The model under review builds one solid part; all positions refer to its coordinate system, in mm. A direction names the side the tool comes from. Give positions to 0.01 mm unless a question says otherwise; leave off trailing zeros. Loops run counter-clockwise (first coordinate to the right, second up) from the corner with the lowest first, then second, coordinate; pieces in that order, holes last. Notation, with made-up numbers: M 12,60 L 27,60 A20 cw 27,73 Z; hole C 29,52 d9. An arc over 180 degrees is marked long. One line per item, written item: value. Start each with the question number.
Q1. We need section C-C on z = -2.75. Write out the cut boundary in (x, y), plus the area to 3 significant figures.
Q2. We need section B-B on x = -21. Write out the cut boundary in (y, z).
Q3. For faces 1 (the face through (-19.8, 7.6, -5)), 2 (the face through (8.834, 10.14, -16.465)), 3 (the face through (15, 10, -10)), 4 (the face through (0, 0, -6)), 5 (the face through (27, 10, -2)), list the 3-axis set-ups (+Z, -Z, +X, -X, +Y, -Y) from which the entire face can be reached by the end or side of a thin tool; tool diameter is ignored.
Q4. We need section D-D on y = 2.5. Write out the cut boundary in (x, z), plus the area to 3 significant figures.
Q5. To check wall thickness, follow line 1 along Y through (x, z) = (21, -2.1); line 2 along X through (y, z) = (11, -4); line 3 along Z through (x, y) = (-19, 15.75). State the ranges of each line that lie inside material, in increasing order. Write a range as from..to.
Q6. We need section A-A on y = 10. Write out the cut boundary in (x, z), plus the area to 3 significant figures.
Q7. Mouldability with a two-part tool opening along X and no side actions: class faces 6 (the face through (11, 10, -16.642)), 7 (the face through (-15, 10, -10)), 8 (the face through (23, 8.5, -2.5)) as released by +X, released by -X, zero draft, split by the parting line, or undercut.
Q8. For pin 1 (2 mm diameter, centred on x = 21.5, y = 13, fed in from -Z); pin 2 (1 mm diameter, centred on x = -8.5, y = 15.5, fed in from -Z); pin 3 (8.5 mm diameter, centred on y = 6, z = -11.5, fed in from +X); pin 4 (10 mm diameter, centred on x = 6.5, y = 15.5, fed in from +Z), all flat-tipped, find the tip position at first contact; note any pin that passes through.
Autodesk Inventor part; units mm, degrees
ref_plane "YZ Plane" through (0, 0, 0) normal (1, 0, 0) x (0, 1, 0)
ref_plane "XZ Plane" through (0, 0, 0) normal (0, 1, 0) x (-1, 0, 0)
ref_plane "XY Plane" through (0, 0, 0) normal (0, 0, 1) x (1, 0, 0)
sketch "Sketch1" plane through (0, 0, 0) normal (0, 1, 0) x (-1, 0, 0)
  circle A0 centre (0, -19.05) radius 9
  line L0 (15, 0) -> (-15, 0)
  line L1 (-15, 0) -> (-15, -16.6415)
  line L2 (-15, -16.6415) -> (15, -16.6415)
  line L3 (15, -16.6415) -> (15, 0)
  line L4 (-27, -5) -> (27, -5)
  line L5 (27, -5) -> (27, 0)
  line L6 (27, 0) -> (-27, 0)
  line L7 (-27, 0) -> (-27, -5)
  line L8 (-27, -5) -> (27, 0) construction
  line L9 (27, -5) -> (-27, 0) construction
  point P0 (0, 0)
  point P1 (0, -2.5)
  point P2 (0, -2.5)
  point P3 (0, -2.5)
  point P4 (15, -5)
  point P5 (15, 0)
  point P6 (-15, -5)
  point P7 (-15, 0)
  point P8 (0, 0)
  dimension "d0" = 18
  dimension "d1" = 19.05
  dimension "d5" = 15
  dimension "d6" = 15
  dimension "d7" = 27
  dimension "d13" = 5
extrude "Extrusion1" add sketch "Sketch1" along normal blind 20 contours A0 L2 L1 L4 L3 | L4 L1 L0 L3 | L3 L6 L5 L4 | L4 L7 L6 L1
sketch "Sketch2" plane through (27, 0, -5) normal (0, 0, -1) x (-1, 0, 0)
  circle A0 centre (6, 10) radius 2.5
  line L0 (0, 0) -> (0, 20)
  line L1 (0, 20) -> (12, 20)
  point P0 (27, 0)
  point P1 (6, 20)
  dimension "d10" = 6
  dimension "d11" = 10
  dimension "d12" = 5
extrude "Extrusion2" cut sketch "Sketch2" against normal through all
mirror "Mirror1" about plane through (0, 0, 0) normal (1, 0, 0) of "Extrusion2"
fillet "Fillet2" radius 1 2 edges at (8.6718, 10, -16.6415) (-8.6718, 10, -16.6415)
fillet "Fillet3" radius 1 2 edges at (27, 10, -5) (-27, 10, -5)
sketch "Sketch3" plane through (-15, 0, -5) normal (0, 0, -1) x (-1, 0, 0)
  circle A0 centre (6, 10) radius 2.5
  circle A1 centre (6, 10) radius 5
  line L0 (11, 20) -> (11, 0)
  point P0 (-15, 0)
fillet "Fillet4" radius 1 2 edges at (15, 10, -5) (-15, 10, -5)
fillet "Fillet5" radius 3 2 edges at (15, 10, -16.6415) (-15, 10, -16.6415)
properties part number "Shaft support"
Solved:
1. outline: M -27,0 L 27,0 L 27,20 L -27,20 Z; hole C -21,10 d5; hole C 21,10 d5
1. area: 1,040 mm2
2. outline: M 0,-5 L 7.5,-5 L 7.5,0 L 0,0 Z; M 12.5,-5 L 20,-5 L 20,0 L 12.5,0 Z
3. face 1: -Z, -X, +Y, -Y
3. face 2: -Z, +Y, -Y
3. face 3: -Z, +X, +Y, -Y
3. face 4: +Z, -Z, +X, -X, -Y
3. face 5: +Z, -Z, +X, +Y, -Y
4. outline: M -27,-4 A1 ccw -26,-5 L -16,-5 A1 cw -15,-6 L -15,-13.64 A3 ccw -12,-16.64 L -9.4,-16.64 A1 ccw -8.46,-15.98 A9 cw 8.46,-15.98 A1 ccw 9.4,-16.64 L 12,-16.64 A3 ccw 15,-13.64 L 15,-6 A1 cw 16,-5 L 26,-5 A1 ccw 27,-4 L 27,0 L -27,0 Z
4. area: 531 mm2
5. line 1: 0..7.5, 12.5..20
5. line 2: -27..-23.29, -18.71..18.71, 23.29..27
5. line 3: -5..0
6. outline: M -27,-4 A1 ccw -26,-5 L -23.5,-5 L -23.5,0 L -27,0 Z; M -18.5,-5 L -16,-5 A1 cw -15,-6 L -15,-13.64 A3 ccw -12,-16.64 L -9.4,-16.64 A1 ccw -8.46,-15.98 A9 cw 8.46,-15.98 A1 ccw 9.4,-16.64 L 12,-16.64 A3 ccw 15,-13.64 L 15,-6 A1 cw 16,-5 L 18.5,-5 L 18.5,0 L -18.5,0 Z; M 23.5,-5 L 26,-5 A1 ccw 27,-4 L 27,0 L 23.5,0 Z
6. area: 481 mm2
7. face 6: zero draft
7. face 7: released by -X
7. face 8: undercut
8. pin 1: z = -5
8. pin 2: z = -16.56
8. pin 3: x = 15
8. pin 4: z = 0
